Design review of the part built by this model. Coordinates are the model's own, in mm. A direction names the side the tool comes from. Coordinates: 2 decimals unless noted, no trailing zeros. Loops run counter-clockwise (first coordinate to the right, second up) from the corner with the lowest first, then second, coordinate; pieces in that order, holes last. Notation, with made-up numbers: (83.25, 32.5) -> (108.25, 32.5) arc R14 cw to (108.25, 38.5) -> close; hole circle Ø9 at (85.25, 36). An arc over 180 degrees is marked (long way). Answer as a JSON object with one key per item and string values.
```python
from build123d import *

# Parameters (mm, degrees)
SKETCH1_W           = 5
SKETCH1_H           = 6
BOSS_EXTRUDE1_DEPTH = 5
SKETCH2_W           = 3.25
SKETCH2_H           = 4.25
CUT_EXTRUDE1_DEPTH  = 5
SKETCH3_R           = 7.5
BOSS_EXTRUDE2_DEPTH = 2


with BuildPart() as part:
    # Sketch1 → Boss-Extrude1 (new body)
    with BuildSketch(Plane(origin=(0, 0, 0), x_dir=(1, 0, 0), z_dir=(0, 1, 0))):
        with Locations((2.5, 3)):
            Rectangle(SKETCH1_W, SKETCH1_H)
    extrude(amount=BOSS_EXTRUDE1_DEPTH)

    # Sketch2 → Cut-Extrude1 (cut)
    with BuildSketch(Plane.XZ):
        with Locations((2.5, -3)):
            Rectangle(SKETCH2_W, SKETCH2_H)
    extrude(amount=-CUT_EXTRUDE1_DEPTH, mode=Mode.SUBTRACT)

    # Sketch3 → Boss-Extrude2 (add)
    with BuildSketch(Plane(origin=(0, 5, 0), x_dir=(1, 0, 0), z_dir=(0, 1, 0))):
        with Locations(Location((2.5, 3, 0), (0, 0, 270))):
            Circle(SKETCH3_R)
    extrude(amount=BOSS_EXTRUDE2_DEPTH)


solid = part.part
```
1) Add section D-D, the plane y = 5.25. Give the boundary of the cut face in (x, z).
Completed:
{"outline": "circle Ø15 at (2.5, -3)"}
2) Add section C-C, the plane x = 2.5. Give the boundary of the cut face in (y, z) (3 decimals), and give its area (4 significant figures).
Completed:
{"outline": "(0, -6) -> (5, -6) -> (5, -10.5) -> (7, -10.5) -> (7, 4.5) -> (5, 4.5) -> (5, 0) -> (0, 0) -> (0, -0.875) -> (5, -0.875) -> (5, -5.125) -> (0, -5.125) -> close", "area": "38.75 mm²"}
3) Add section A-A, the plane y = 3. Give the boundary of the cut face in (x, z) (3 decimals), and give its area (3 significant figures).
Completed:
{"outline": "(0, -6) -> (5, -6) -> (5, 0) -> (0, 0) -> close; hole (0.875, -5.125) -> (4.125, -5.125) -> (4.125, -0.875) -> (0.875, -0.875) -> close", "area": "16.2 mm²"}
4) Clearance check with flat-ended pins moving along their axes: pin 1 Ø1 at (x, z) = (-2.5, -0.5) entering from -Y; pin 2 Ø1.5 at (y, z) = (5, -8.5) entering from -X; pin 3 Ø2 at (y, z) = (1.5, -2) entering from +X; pin 4 Ø4 at (x, y) = (3.5, 3.5) entering from +Z. State where each tip first meets the part, or that it passes through.
Completed:
{"pin 1": "y = 5", "pin 2": "x = -3.3", "pin 3": "x = 5", "pin 4": "z = 4.5"}
5) Wall thickness on probe 1 along Z at (x, y) = (2.5, 3) (3 decimals); probe 2 along X at (y, z) = (3.75, -2.75) (3 decimals); probe 3 along Y at (x, z) = (5.75, -3.75): over which ranges is each line inside the solid? List them lowest first.
Completed:
{"probe 1": "-6 to -5.125, -0.875 to 0", "probe 2": "0 to 0.875, 4.125 to 5", "probe 3": "5 to 7"}
6) The part is to be moulded in two halves that separate along Z. For faces 1 (the flat face through (2, 2, 0)), 2 (the flat face through (2, 2, -0.875)), 3 (the flat face through (2.6, 5, 0.2)), say which applies: pulls with the +Z half, pulls with the -Z half, needs draft (parallel to the pull), parting line crosses it, or undercut.
Completed:
{"face 1": "pulls with the +Z half", "face 2": "undercut", "face 3": "needs draft"}
7) For faces 4 (the flat face through (2, 2, -6)), 5 (the flat face through (0.875, 2, -3)), 6 (the flat face through (5, 2, -3)), 7 (the flat face through (0, 2, -3)), 8 (the cylindrical face through (8.824, 5.986, 1.032)), list the 3-axis set-ups (+Z, -Z, +X, -X, +Y, -Y) from which the entire face can be reached by the end or side of a thin tool; tool diameter is ignored.
Completed:
{"face 4": "-Z, +X, -X, -Y", "face 5": "-Y", "face 6": "+Z, -Z, +X, -Y", "face 7": "+Z, -Z, -X, -Y", "face 8": "+Y, -Y"}
8) Add section B-B, the plane z = -3. Give the boundary of the cut face in (x, y) (3 decimals), and give its area (4 significant figures).
Completed:
{"outline": "(-5, 5) -> (0, 5) -> (0, 0) -> (0.875, 0) -> (0.875, 5) -> (4.125, 5) -> (4.125, 0) -> (5, 0) -> (5, 5) -> (10, 5) -> (10, 7) -> (-5, 7) -> close", "area": "38.75 mm²"}
